Autodesk Inventor part; units mm, degrees
ref_plane "YZ Plane" through (0, 0, 0) normal (1, 0, 0) x (0, 1, 0)
ref_plane "XZ Plane" through (0, 0, 0) normal (0, 1, 0) x (-1, 0, 0)
ref_plane "XY Plane" through (0, 0, 0) normal (0, 0, 1) x (1, 0, 0)
sketch "Sketch1" plane through (0, 0, 0) normal (0, 1, 0) x (-1, 0, 0)
  circle A0 centre (0, 0) radius 2.5
  circle A1 centre (-27.7848, -0.0003) radius 2.5
  circle A2 centre (-34.6699, 23.8458) radius 2.5
  circle A3 centre (-20.1174, 31.2789) radius 2.5
  line L0 (-32.1699, 23.8458) -> (-25.2848, -0.0003)
  line L1 (-37.1699, 23.8458) -> (-30.1893, -0.6845)
  line L2 (-27.9447, 2.4946) -> (-0.0005, 2.5)
  line L3 (-0.0005, -2.5) -> (-27.7848, -2.5003)
  line L4 (-19.1471, 28.9749) -> (-33.5318, 21.6199)
  arc A4 (-33.5318, 21.6199) -> (-35.8061, 26.0727) centre (-34.6699, 23.8458) ccw
  line L5 (-21.4171, 33.4145) -> (-35.8061, 26.0727)
  dimension "d0" = 5
  dimension "d1" = 5
  dimension "d2" = 5
  dimension "d3" = 5
extrude "Extrusion1" add sketch "Sketch1" along normal blind 3 contours A0 | A0 L3 A1 L0 L2 | L0 A1 L1 A2 L4 | A1 L0 | L4 A2 L0 | L0 A2 L5 A3 L4 | A1 L0 | A2 L1 | A3 picked at (-35.4421, 23.1763)
sketch "Sketch2" plane through (0, 0, 0) normal (0, -1, 0) x (1, 0, 0)
  circle A0 centre (0, 0) radius 1.4
  dimension "d6" = 2.8
extrude "Extrusion2" cut sketch "Sketch2" against normal blind 8
thread "Thread2"
sketch "Sketch3" plane through (0, 0, 0) normal (0, -1, 0) x (1, 0, 0)
  arc A0 (21.4171, 33.4145) -> (19.1471, 28.9749) centre (20.1174, 31.2789) ccw
  circle A1 centre (20.1174, 31.2789) radius 1.5
  point P0 (0, 0)
  dimension "d13" = 3
extrude "Extrusion3" cut sketch "Sketch3" against normal blind 10
thread "Thread3"
properties part number "Servo_Arm_Hook_F_new"
Can you work these out from the model? Positions are in its coordinate system, mm. A direction names the side the tool comes from. Round coordinates to 2 decimals unless told otherwise and drop trailing zeros. Loops run counter-clockwise (first coordinate to the right, second up) from the corner with the lowest first, then second, coordinate; pieces in that order, holes last. Notation, with made-up numbers: (83.5, 67.5) - (91.5, 67.5) arc R22 cw to (91.5, 99.5) - close; hole circle Ø8 at (-32, 74.5). An arc over 180 degrees is marked (long way). Write item = value, one per line. Start each with the question number.
(1) If we section it at A-A (z = 0): Please give me the cut outline in (x, y), and give its area (3 significant figures).
(2) For P1, Ø1.5, axis at y = 2.5, z = 10, coming from the +X side; P2, Ø0.9, axis at x = 18, y = 1.5, coming from the +Z side, each with a flat end and sliding along its axis, tell me the tip position at first contact or that it passes through.
(3) If we section it at B-B (x = 27): Please give me the cut outline in (y, z).
(4) If we section it at D-D (y = 1.2): Please give me the cut outline in (x, z), and give its area (3 significant figures).
(5) If we mould it in two halves opening along X, with no side actions, what happens to faces 3 (the face through (17.92, 1.48, 32.47)), 4 (the face through (36.81, 1.48, 25.14)), 5 (the face through (21.55, 1.48, 31.73)), 6 (the face through (-1.4, 1.48, 0.06))? For each: released by +X, released by -X, zero draft, split by the parting line, or undercut.
(6) For faces 1 (the face through (29, 3, 12)), 2 (the face through (25.38, 1.48, 25.79)), which set-ups out of +Z, -Z, +X, -X, +Y, -Y let a thin tool reach every point of the face, with its end or its side?
(7) If I drill on probe 1 along Z at (x, y) = (16.5, 1.6); probe 2 along Z at (x, y) = (0, 1.75); probe 3 along Z at (x, y) = (20.5, 0.3), over which ranges is the centre line in solid material (lowest first)? Write a range as [from, to].
(8) If we section it at C-C (x = 20): Please give me the cut outline in (y, z).
Ans:
q1.outline = (-2.5, 0) - (-1.4, 0) - (-1.4, 3) - (-2.5, 3) - close; (1.4, 0) - (30.38, 0) - (30.38, 3) - (1.4, 3) - close
q1.area = 90.3 mm²
q2.P1 = 33.44
q2.P2 = 33.14
q3.outline = (0, -2.5) - (3, -2.5) - (3, 5.94) - (0, 5.94) - close; (0, 24.96) - (3, 24.96) - (3, 30.57) - (0, 30.57) - close
q4.outline = (0, -2.5) - (27.78, -2.5) arc R2.5 ccw to (30.19, -0.68) - (37.17, 23.85) arc R2.5 ccw to (35.81, 26.07) - (21.42, 33.41) arc R2.5 ccw (long way) to (19.15, 28.97) - (31.79, 22.51) - (26.01, 2.49) - (0, 2.5) arc R2.5 ccw to start; hole circle Ø2.8 at (0, 0); hole circle Ø3 at (20.12, 31.28)
q4.area = 346 mm²
q5.face_3 = split by the parting line
q5.face_4 = released by +X
q5.face_5 = undercut
q5.face_6 = undercut
q6.face_1 = +Z, -Z, +X, -X, +Y
q6.face_2 = -X, +Y, -Y
q7.probe_1 = [-2.5, 2.5]
q7.probe_2 = [-2.5, -1.4], [1.4, 2.5]
q7.probe_3 = [-2.5, 2.5], [28.28, 29.83], [32.73, 33.75]
q8.outline = (0, -2.5) - (3, -2.5) - (3, 2.5) - (0, 2.5) - close; (0, 28.54) - (3, 28.54) - (3, 29.78) - (0, 29.78) - close; (0, 32.77) - (3, 32.77) - (3, 33.78) - (0, 33.78) - close
